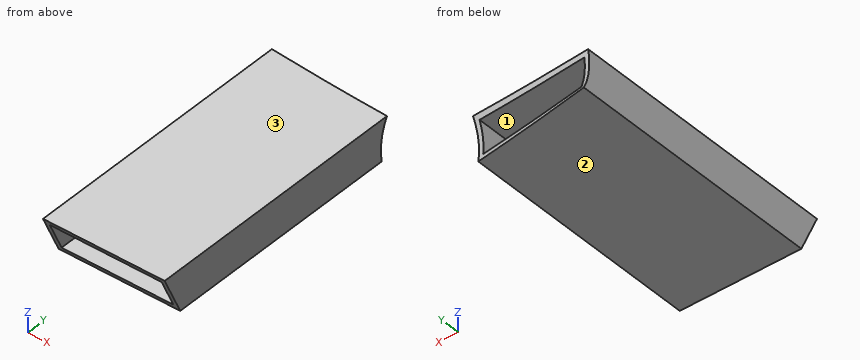
from build123d import *

# Parameters (mm, degrees)
SKETCH1_W           = 76.2
SKETCH1_H           = 25.4
SKETCH1_W_2         = 70.104
SKETCH1_H_2         = 19.304
BOSS_EXTRUDE1_DEPTH = 200
SKETCH3_W           = 76.2
SKETCH3_H           = 25.4
SKETCH3_W_2         = 70.104
SKETCH3_H_2         = 19.304
BOSS_EXTRUDE2_DEPTH = 38.1
CUT_EXTRUDE1_DEPTH  = 77.2
CUT_EXTRUDE5_START  = 13.832764
SKETCH7_R           = 38.1
CUT_EXTRUDE5_DEPTH  = 83.124802


with BuildPart() as part:
    # Sketch1 → Boss-Extrude1 (new body)
    with BuildSketch(Plane(origin=(0, 0, 0), x_dir=(1, 0, 0), z_dir=(0, 1, 0))):
        Rectangle(SKETCH1_W, SKETCH1_H)
        Rectangle(SKETCH1_W_2, SKETCH1_H_2, mode=Mode.SUBTRACT)
    extrude(amount=BOSS_EXTRUDE1_DEPTH)

    # Sketch3 → Boss-Extrude2 (add)
    with BuildSketch(Plane.XZ):
        Rectangle(SKETCH3_W, SKETCH3_H)
        Rectangle(SKETCH3_W_2, SKETCH3_H_2, mode=Mode.SUBTRACT)
    extrude(amount=BOSS_EXTRUDE2_DEPTH)

    # Sketch4 → Cut-Extrude1 (cut, through all)
    with BuildSketch(Plane(origin=(38.1, 0, 0), x_dir=(0, 0, -1), z_dir=(1, 0, 0))):
        Polygon((-18.94463971, -8.788530579), (21.02313948, 9.752758934), (26.07322677, -49.294265894), (-15.918593218, -47.517542491), align=None)
    extrude(amount=-CUT_EXTRUDE1_DEPTH, mode=Mode.SUBTRACT)

    # Sketch7 → Cut-Extrude5 (cut)
    with BuildSketch(Plane(origin=(56.875227758, 193.523427606, -7.656864493), x_dir=(0.131571603, -0.016382038, 0.991171298), z_dir=(-0.984807753, 0.112143352, 0.132580384)).offset(CUT_EXTRUDE5_START)):
        Circle(SKETCH7_R)
    extrude(amount=CUT_EXTRUDE5_DEPTH, mode=Mode.SUBTRACT)


solid = part.part
Input: part model. Units: mm. Frame: model coordinates. Face numbers are marked on the shaded views. Give positions to 0.01 mm unless a question says otherwise; leave off trailing zeros. Order: outer loops, then holes, each group sorted by start corner. A loop starts at its lowest first (then second) coordinate and runs counter-clockwise, first axis right, second up. Notation, with made-up numbers: (85, 72) - (98, 72) arc R15 cw to (98, 79) - close; hole circle Ø8 at (21.25, 61). An arc over 180 degrees is marked (long way). Answer as a JSON object with one key per item and string values. Group by question number.
Q1. Line query: probe 1 along Z at (x, y) = (-13.5, 94); probe 2 along X at (y, z) = (11, -4); probe 3 along Y at (x, z) = (-11, 11.25). Output: solid intervals per line, ascending.
Q2. First-contact query: pin 1 Ø1.5 at (x, z) = (-27.5, 10) entering from -Y. Flat tip, straight axial feed; report the tip coordinate or a pass-through.
Q3. Mould query, pull axis Z, two halves, no side actions, for the marked faces 1, 2 and 3. Classes: pulls with the +Z half, pulls with the -Z half, needs draft (parallel to the pull), parting line crosses it, or undercut.
Q4. Cut plane A-A, the plane y = 62. Output: boundary loops of the cut face in (x, z), then the cut area to 3 significant figures.
Results:
{
 "1": {"probe 1": "-12.7 to -9.65, 9.65 to 12.7", "probe 2": "-38.1 to -35.05, 35.05 to 38.1", "probe 3": "-5.22 to 164.32"},
 "2": {"pin 1": "y = -4.99"},
 "3": {"face 1": "undercut", "face 2": "pulls with the -Z half", "face 3": "pulls with the +Z half"},
 "4": {"outline": "(-38.1, -12.7) - (38.1, -12.7) - (38.1, 12.7) - (-38.1, 12.7) - close; hole (-35.05, -9.65) - (35.05, -9.65) - (35.05, 9.65) - (-35.05, 9.65) - close", "area": "582 mm^2"}
}
